Source: CAD feature listing. Evaluate the final solid. Frame: model axes, mm. Face numbers are marked on the shaded views. Round coordinates to 2 decimals unless told otherwise and drop trailing zeros. Write each loop counter-clockwise with the first axis right and the second up, starting at its lowest first coordinate (ties: lowest second). Pieces come first, ordered by that corner, then holes. Notation, with made-up numbers: M 89.5,56 L 111.5,56 A19 ccw 111.5,87 Z; hole C 74,57.5 d4. An arc over 180 degrees is marked long. Answer in a Markdown table with one row per item.
from build123d import *

# Parameters (mm, degrees)
FILLET1_R = 0.635


with BuildPart() as part:
    # Sketch1 → Revolve1 (revolve)
    with BuildSketch(Plane.XY, mode=Mode.PRIVATE) as revolve1_sk:
        with BuildLine():
            Line((-23.425738216, 5.85380266), (-21.393738216, 5.85380266))
            Line((-21.393738216, 5.85380266), (-19.996738216, 4.45680266))
            Line((-19.996738216, 4.45680266), (-18.599738216, 5.85380266))
            Line((-18.599738216, 5.85380266), (-17.964738216, 5.85380266))
            Line((-17.964738216, 5.85380266), (-17.964738216, 7.17460266))
            Line((-17.964738216, 7.17460266), (-18.980738216, 7.17460266))
            ThreePointArc((-18.980738216, 7.17460266), (-19.996738216, 8.19060266), (-21.012738216, 7.17460266))
            Line((-21.012738216, 7.17460266), (-21.393738216, 7.17460266))
            Line((-21.393738216, 7.17460266), (-21.393738216, 9.07960266))
            Line((-21.393738216, 9.07960266), (-17.329738216, 9.07960266))
            Line((-17.329738216, 9.07960266), (-17.329738216, 10.98460266))
            Line((-17.329738216, 10.98460266), (-23.425738216, 10.98460266))
            Line((-23.425738216, 10.98460266), (-23.425738216, 9.07960266))
            Line((-23.425738216, 9.07960266), (-23.425738216, 5.85380266))
        make_face()
    revolve(revolve1_sk.sketch.rotate(Axis((-23.425738216, -8.06539734, 0), (1, 0, 0)), 90), axis=Axis((-23.425738216, -8.06539734, 0), (1, 0, 0)))

    # Fillet1
    fillet1_edges = [part.edges().sort_by_distance(p)[0] for p in [
        (-17.329738216, -8.06539734, -19.05),
        (-23.425738216, -8.06539734, -19.05),
    ]]
    fillet(fillet1_edges, radius=FILLET1_R)


solid = part.part
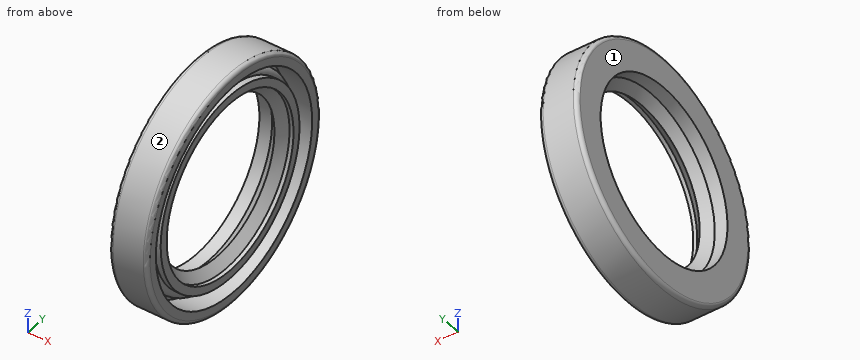
Q1. Material intervals for probe 1 along Y at (x, z) = (-18.3, 0); probe 2 along Y at (x, z) = (-21.25, 2); probe 3 along Z at (x, y) = (-21.25, -15.5), sorted ascending.
Solutions:
| item | result |
|---|---|
| probe 1 | y = -27.12 to -25.21, -23.31 to -21.98, 5.85 to 7.17, 9.08 to 10.98 |
| probe 2 | y = -27.01 to -25.09, -23.17 to -21.69, 5.56 to 7.04, 8.96 to 10.88 |
| probe 3 | z = -17.54 to -15.45, -13.3 to -11.6, 11.6 to 13.3, 15.45 to 17.54 |
Q2. Contact query for flat-ended pins moving along their axis: pin 1 Ø10.5 at (y, z) = (-1.5, -6.5) entering from +X; pin 2 Ø1.5 at (x, y) = (-18, -9) entering from +Z; pin 3 Ø1.5 at (x, z) = (-20.5, -14) entering from +Y. Output: stop coordinate, or through.
Solutions:
| item | result |
|---|---|
| pin 1 | stops at x = -17.96 |
| pin 2 | stops at z = 19.05 |
| pin 3 | stops at y = 5.62 |
Q3. Section B-B (x = -22). Return loops of the section in (y, z).
Solutions:
| item | result |
|---|---|
| outline | C -8.07,0 d38.1; hole C -8.07,0 d27.84 |
Q4. Pull-direction query (Y, two-part tool) for the marked faces 1 and 2; classes: pulls with the +Y half, pulls with the -Y half, needs draft (parallel to the pull), parting line crosses it, or undercut.
Solutions:
| item | result |
|---|---|
| face 1 | needs draft |
| face 2 | parting line crosses it |
